from build123d import *

# Parameters (mm, degrees)
SKETCH2_R               = 27.5
SKETCH2_R_2             = 22.5
BOSS_EXTRUDE2_DEPTH     = 15
SKETCH3_R               = 35
BOSS_EXTRUDE3_DEPTH     = 10
SKETCH4_R               = 22.5
CUT_EXTRUDE1_DEPTH      = 31
CUT_EXTRUDE1_DEPTH_BACK = 11


with BuildPart() as part:
    # Sketch2 → Boss-Extrude2 (new body, symmetric)
    with BuildSketch(Plane.XY):
        Circle(SKETCH2_R)
        Circle(SKETCH2_R_2, mode=Mode.SUBTRACT)
    extrude(amount=BOSS_EXTRUDE2_DEPTH, both=True)

    # Sketch3 → Boss-Extrude3 (add)
    with BuildSketch(Plane.XY.offset(15)):
        Circle(SKETCH3_R)
    extrude(amount=BOSS_EXTRUDE3_DEPTH)

    # Sketch4 → Cut-Extrude1 (cut, two sides)
    with BuildSketch(Plane(origin=(0, 0, 15), x_dir=(-1, 0, 0), z_dir=(0, 0, -1))) as cut_extrude1_sk:
        Circle(SKETCH4_R)
    extrude(amount=CUT_EXTRUDE1_DEPTH, mode=Mode.SUBTRACT)
    extrude(cut_extrude1_sk.sketch, amount=-CUT_EXTRUDE1_DEPTH_BACK, mode=Mode.SUBTRACT)


solid = part.part
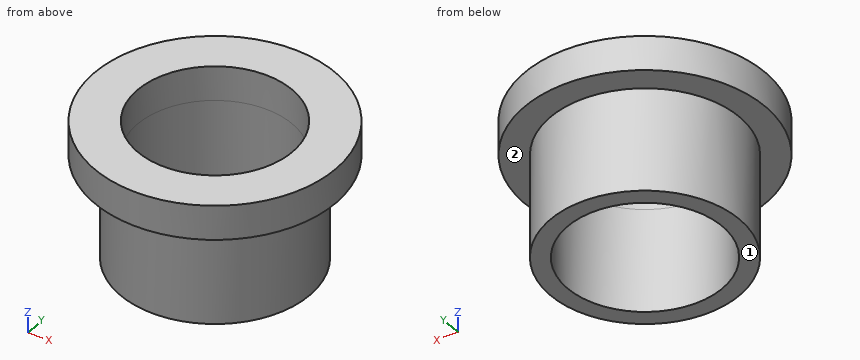
Read the model definition and answer for the solid it produces. Units are mm, in the model's axes. Face numbers are marked on the shaded views. A direction names the side the tool comes from. Give positions to 0.01 mm unless a question says otherwise; leave off trailing zeros. Write each loop counter-clockwise with the first axis right and the second up, starting at its lowest first coordinate (ties: lowest second). Pieces come first, ordered by that corner, then holes. Notation, with made-up numbers: M 81,3.25 L 139,3.25 A29 cw 139,23.25 Z; hole C 35,72 d8. An arc over 180 degrees is marked long. One line per item, written item: value. Start each with the question number.
(1) Find section A-A (x = 0). Determine the outline of the cut face in (y, z), plus the area to 3 significant figures.
(2) Find section C-C (z = 7). Determine the outline of the cut face in (x, y).
(3) Find the intervals of material crossed by line 1 (Y direction, x = 0, z = 20); line 2 (Y direction, x = 0, z = -5); line 3 (X direction, y = -12, z = -5.5), in increasing order.
(4) Flat-ended cylindrical pins translate along their axes: pin 1 Ø8 at (x, z) = (-16, 3) entering from -Y; pin 2 Ø1 at (y, z) = (18.5, 18.5) entering from +X; pin 3 Ø8 at (x, z) = (-8, -8.5) entering from +Y. Find the tip coordinate at first contact, or state that the pin passes through.
(5) A tool of negligible diameter and unlimited length cuts with its end or side. For the marked faces 1 and 2, from which of +Z, -Z, +X, -X, +Y, -Y can it reach the whole face along a straight path? Write none if from no direction.
(6) Find section D-D (y = -26.5). Determine the outline of the cut face in (x, z), plus the area to 3 significant figures.
Results below:
1. outline: M -35,15 L -27.5,15 L -27.5,-15 L -22.5,-15 L -22.5,25 L -35,25 Z; M 22.5,-15 L 27.5,-15 L 27.5,15 L 35,15 L 35,25 L 22.5,25 Z
1. area: 550 mm^2
2. outline: C 0,0 d55; hole C 0,0 d45
3. line 1: y = -35 to -22.5, 22.5 to 35
3. line 2: y = -27.5 to -22.5, 22.5 to 27.5
3. line 3: x = -24.74 to -19.03, 19.03 to 24.74
4. pin 1: stops at y = -24.74
4. pin 2: stops at x = 30.02
4. pin 3: stops at y = 27.21
5. face 1: -Z, +X, -X, +Y, -Y
5. face 2: -Z
6. outline: M -22.86,15 L -7.35,15 L -7.35,-15 L 7.35,-15 L 7.35,15 L 22.86,15 L 22.86,25 L -22.86,25 Z
6. area: 898 mm^2
